Autodesk Inventor part; units mm, degrees
ref_plane "YZ Plane" through (0, 0, 0) normal (1, 0, 0) x (0, 1, 0)
ref_plane "XZ Plane" through (0, 0, 0) normal (0, 1, 0) x (-1, 0, 0)
ref_plane "XY Plane" through (0, 0, 0) normal (0, 0, 1) x (1, 0, 0)
sketch "Sketch1" plane through (0, 0, 0) normal (0, 1, 0) x (-1, 0, 0)
  line L0 (5.1091, 27.5) -> (-62.3909, 27.5)
  line L1 (-62.3909, 27.5) -> (-62.3909, -15)
  line L2 (-62.3909, -15) -> (5.1091, -15)
  line L3 (5.1091, -15) -> (5.1091, 27.5)
  line L4 (5.1091, 6.25) -> (-62.3909, 6.25)
  point P0 (0, 0)
  dimension "d0" = 42.5
  dimension "d1" = 67.5
extrude "Extrusion1" add sketch "Sketch1" along normal blind 5.31
sketch "Sketch2" plane through (0, 5.31, 0) normal (0, 1, 0) x (1, 0, 0)
  circle A0 centre (9.9709, -6.25) radius 0.5
  circle A1 centre (15.6009, -13.28) radius 0.5
  circle A2 centre (15.6009, 0.78) radius 0.5
  circle A3 centre (47.3109, -6.25) radius 0.5
  line L0 (-5.1091, -6.25) -> (62.3909, -6.25) construction
  line L1 (15.6009, 15.6122) -> (15.6009, -24.3614) construction
  line L2 (11.4709, -11.78) -> (45.8109, -11.78)
  line L3 (45.8109, -11.78) -> (45.8109, -0.72)
  line L4 (45.8109, -0.72) -> (11.4709, -0.72)
  line L5 (11.4709, -0.72) -> (11.4709, -11.78)
  circle A4 centre (-0.8591, 10.75) radius 1.625
  line L6 (62.3909, 15) -> (-5.1091, 15)
  circle A5 centre (-0.8591, -23.25) radius 1.625
  line L7 (-5.1091, -27.5) -> (62.3909, -27.5)
  circle A6 centre (58.1409, 10.75) radius 1.625
  circle A7 centre (58.1409, -23.25) radius 1.625
  line L8 (62.3909, -27.3764) -> (62.3909, 12.6236)
  line L9 (28.6409, -27.5) -> (28.6409, 15) construction
  line L10 (62.3909, -27.5) -> (62.3909, 15)
  line L11 (-5.1091, -27.5) -> (62.3909, -27.5)
  line L12 (-5.1091, 15) -> (-5.1091, -27.5)
  line L13 (62.3909, 15) -> (-5.1091, 15)
  point P0 (0, 0)
  dimension "d4" = 1
  dimension "d15" = 14.06
  dimension "d23" = 37.34
  dimension "d39" = 5.63
  dimension "d70" = 4.25
  dimension "d79" = 3.25
  dimension "d82" = 1
  dimension "d83" = 1
  dimension "d84" = 1
  dimension "d85" = 1
  dimension "d90" = 4.25
  dimension "d91" = 4.25
  dimension "d93" = 34
  dimension "d94" = 59
  dimension "d100" = 11.06
extrude "Extrusion2" cut sketch "Sketch2" against normal through all contours A0 | A1 | A2 | A3 | L5 L4 L3 L2 | A4 | A5 | A6 | A7
sketch "Sketch4" plane through (0, 5.31, 0) normal (0, 1, 0) x (1, 0, 0)
  circle A0 centre (-0.8591, 10.75) radius 3.625
  circle A1 centre (58.1409, -23.25) radius 3.625
  circle A2 centre (58.1409, 10.75) radius 3.625
  circle A3 centre (-0.8591, -23.25) radius 3.625
  circle A4 centre (-0.8591, -23.25) radius 1.625 construction
  circle A5 centre (58.1409, -23.25) radius 1.625 construction
  circle A6 centre (-0.8591, 10.75) radius 1.625 construction
  circle A7 centre (58.1409, 10.75) radius 1.625 construction
  circle A8 centre (58.1409, -23.25) radius 1.625
  circle A9 centre (-0.8591, -23.25) radius 1.625
  circle A10 centre (-0.8591, 10.75) radius 1.625
  circle A11 centre (58.1409, 10.75) radius 1.625
  circle A12 centre (47.8109, -13.78) radius 1
  circle A13 centre (9.4709, -13.78) radius 1
  circle A14 centre (47.8109, 1.28) radius 1
  circle A15 centre (9.4709, 1.28) radius 1
  line L0 (45.8109, -11.78) -> (11.4709, -11.78)
  line L1 (45.8109, -0.72) -> (45.8109, -11.78)
  line L2 (28.6409, -33.9575) -> (28.6409, 25.5773) construction
  line L3 (71.7292, -6.25) -> (-26.8251, -6.25) construction
  line L4 (47.8109, -13.78) -> (9.4709, -13.78) construction
  line L5 (47.8109, 1.28) -> (9.4709, 1.28) construction
  circle A16 centre (28.6409, 1.28) radius 1
  circle A17 centre (28.6409, -13.78) radius 1
  point P0 (0, 0)
  point P1 (56.8909, 12)
  point P2 (-2.1091, 12)
  dimension "d92" = 2
  dimension "d95" = 2
  dimension "d96" = 2
  dimension "d97" = 2
extrude "Extrusion4" add sketch "Sketch4" along normal blind 2
sketch "Sketch5" plane through (58.1409, 7.31, -10.75) normal (0, 1, 0) x (1, 0, 0)
  circle A0 centre (0, -34) radius 1.625
  circle A1 centre (0, -34) radius 1
  circle A2 centre (0, -34) radius 3.625
  circle A3 centre (-59, -34) radius 1.625
  circle A4 centre (-59, -34) radius 1.625
  circle A5 centre (-59, -34) radius 3.625
  circle A6 centre (-59, -34) radius 1.625
  circle A7 centre (-59, -34) radius 3.625
  circle A8 centre (0, -34) radius 3.625
  circle A9 centre (-59, 0) radius 1.625
  circle A10 centre (0, 0) radius 1.625
  circle A11 centre (-59, 0) radius 3.625
  circle A12 centre (0, 0) radius 3.625
  circle A13 centre (0, 0) radius 3.625
  circle A14 centre (0, 0) radius 1.625
  circle A15 centre (-59, 0) radius 1.625
  circle A16 centre (-59, 0) radius 3.625
  point P0 (-58.1409, -10.75)
extrude "Extrusion5" add sketch "Sketch5" along normal blind 2.3 contours A2 | A5 | A11 | A12
equation "\"d31\" = d69"
properties part number "490HV_MicrofluidicClamp"
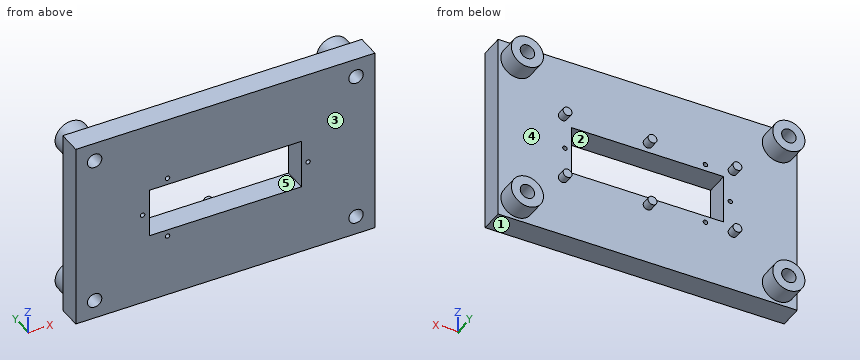
CAD build for the part. Positions are in the model's coordinates, mm. Face numbers are marked on the shaded views. A direction names the side the tool comes from. Give positions to 0.01 mm unless a question says otherwise; leave off trailing zeros. Order: outer loops, then holes, each group sorted by start corner. A loop starts at its lowest first (then second) coordinate and runs counter-clockwise, first axis right, second up. Notation, with made-up numbers: M 2.25,10.5 L 39.25,10.5 A22 cw 39.25,19.5 Z; hole C -39.75,89 d9. An arc over 180 degrees is marked long. Put each result on its own line as item: value. Start each with the question number.
(1) Mould opens along X. For the marked faces 3, 4 and 5 say: +X half, -X half, draft (parallel to the pull), parting line (faces both ways), or undercut.
(2) Saw through at B-B, the plane x = 36.5. Write the cut outline in (y, z), then the cut area to 3 significant figures.
(3) Which spindle directions (+Z, -Z, +X, -X, +Y, -Y) get a long thin tool onto all of the face, cutting with end or side? Do the marked faces 1 and 2. Say none if no direction does.
(4) Flat gauge pins, fed straight in: pin 1 Ø5 at (x, z) = (58.14, -10.75) entering from -Y; pin 2 Ø4 at (x, z) = (5, 17) entering from +Y; pin 3 Ø0.6 at (x, z) = (10, 14.5) entering from +Y. Where does each tip first touch, or does it go through?
(5) Saw through at C-C, the plane z = -10.75. Write the cut outline in (x, y).
(6) Saw through at A-A, the plane y = 6.25. Give the number of separate pieces and of enclosed holes in the cut face, then the cut area to 3 significant figures.
(7) Saw through at D-D, the plane z = 2.5. Write the cut outline in (x, y).
(8) Drill centre lines: line 1 along X through (y, z) = (2.1, 6.25); line 2 along Z through (x, y) = (28.5, 2); line 3 along Z through (x, y) = (-0.5, 5.5). Where is each one in solid material? Low to high.
Check result:
1. face 3: draft
1. face 4: undercut
1. face 5: undercut
2. outline: M 0,-15 L 5.31,-15 L 5.31,0.72 L 0,0.72 Z; M 0,11.78 L 5.31,11.78 L 5.31,27.5 L 0,27.5 Z
2. area: 167 mm2
3. face 1: -Z, +X, -X, +Y, -Y
3. face 2: +Y, -Y
4. pin 1: stops at y = 0
4. pin 2: stops at y = 5.31
4. pin 3: stops at y = 7.31
5. outline: M -5.11,0 L -2.48,0 L -2.48,9.61 L -4.48,9.61 L -4.48,5.31 L -5.11,5.31 Z; M 0.77,0 L 56.52,0 L 56.52,9.61 L 54.52,9.61 L 54.52,5.31 L 2.77,5.31 L 2.77,9.61 L 0.77,9.61 Z; M 59.77,0 L 62.39,0 L 62.39,5.31 L 61.77,5.31 L 61.77,9.61 L 59.77,9.61 Z
6. separate pieces: 10
6. enclosed holes: 4
6. area: 151 mm2
7. outline: M -5.11,0 L 11.47,0 L 11.47,5.31 L -5.11,5.31 Z; M 45.81,0 L 62.39,0 L 62.39,5.31 L 45.81,5.31 Z
8. line 1: x = -5.11 to 9.47, 10.47 to 11.47, 45.81 to 46.81, 47.81 to 62.39
8. line 2: z = -15 to 0.72, 11.78 to 27.5
8. line 3: z = -14.36 to -12.33, -9.17 to -7.14, 19.64 to 21.67, 24.83 to 26.86
